Could you check a few things on this drawing? It's one solid part, dimensions in mm from its lowest x, y, z. A direction names the side the tool comes from. Round coordinates to 2 decimals unless told otherwise and drop trailing zeros. Write each loop counter-clockwise with the first axis right and the second up, starting at its lowest first coordinate (ties: lowest second). Pieces come first, ordered by that corner, then holes. Notation, with made-up numbers: M 36,20.25 L 85,20.25 A6 ccw 85,31.25 Z; hole C 7.25,-38 d4. An arc over 180 degrees is marked long. One line per question, with ' | ' between items. Start each with the question number.
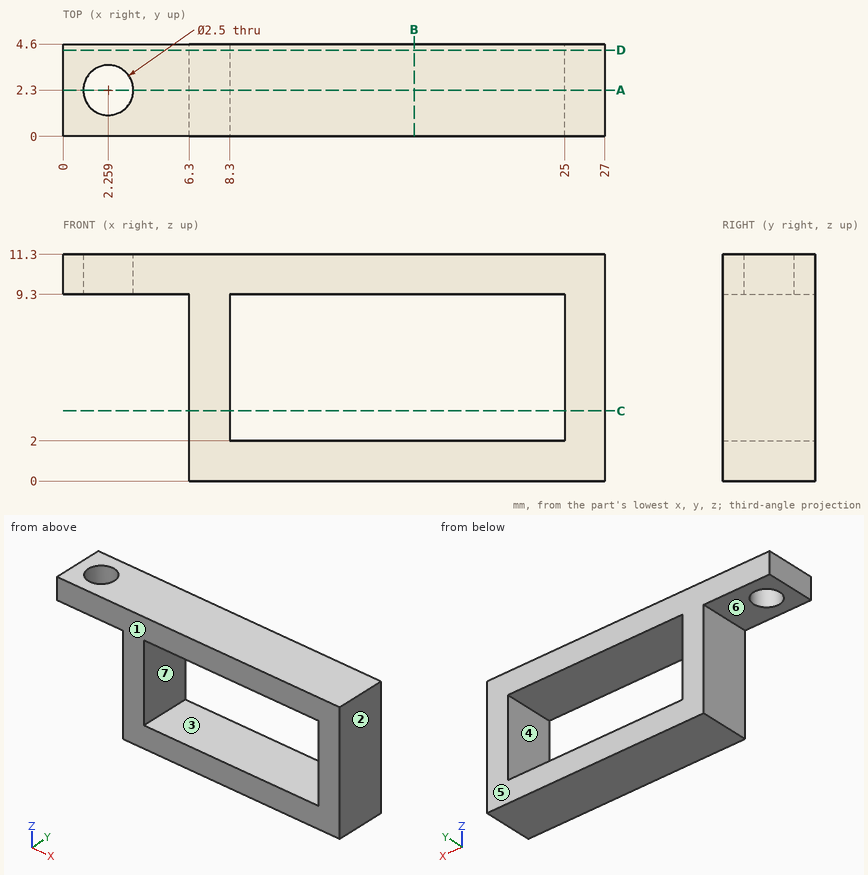
1. If we mould it in two halves opening along X, with no side actions, what happens to the marked faces 1, 2, 3 and 4? For each: released by +X, released by -X, zero draft, split by the parting line, or undercut.
2. I need wall thicknesses on line 1 along X through (y, z) = (3.05, 2.25); line 2 along Z through (x, y) = (19, 3.95); line 3 along Z through (x, y) = (4.5, 0.4). Which ranges of each line are inside material? Lowest first, please. Write a range as from..to.
3. Suppose I cut it at A-A (y = 2.3). Write out the boundary of the cut face in (x, z), and give its area (3 significant figures).
4. Suppose I cut it at B-B (x = 17.5). Write out the boundary of the cut face in (y, z).
5. Which directions (+Z, -Z, +X, -X, +Y, -Y) give clear straight access to the entire face, cutting with the end or side of a thin tool? Please do the marked faces 5, 6 and 7.
6. Suppose I cut it at C-C (z = 3.5). Write out the boundary of the cut face in (x, y).
7. Suppose I cut it at D-D (y = 4.3). Write out the boundary of the cut face in (x, z).
Computed:
1) face 1: zero draft | face 2: released by +X | face 3: undercut | face 4: undercut
2) line 1: x = 6.3..8.3, 25..27 | line 2: z = 0..2, 9.3..11.3 | line 3: z = 9.3..11.3
3) outline: M 0,9.3 L 1.01,9.3 L 1.01,11.3 L 0,11.3 Z; M 3.51,9.3 L 6.3,9.3 L 6.3,0 L 27,0 L 27,11.3 L 3.51,11.3 Z; hole M 8.3,2 L 25,2 L 25,9.3 L 8.3,9.3 Z | area: 120 mm²
4) outline: M 0,0 L 4.6,0 L 4.6,2 L 0,2 Z; M 0,9.3 L 4.6,9.3 L 4.6,11.3 L 0,11.3 Z
5) face 5: +Z, -Z, +X, -X, +Y | face 6: -Z, -X, +Y, -Y | face 7: +Y, -Y
6) outline: M 6.3,0 L 8.3,0 L 8.3,4.6 L 6.3,4.6 Z; M 25,0 L 27,0 L 27,4.6 L 25,4.6 Z
7) outline: M 0,9.3 L 6.3,9.3 L 6.3,0 L 27,0 L 27,11.3 L 0,11.3 Z; hole M 8.3,2 L 25,2 L 25,9.3 L 8.3,9.3 Z
